Geometry: see drawing. Coordinates: mm, zero at the bounding-box minimum. Coordinates: 2 decimals unless noted, no trailing zeros. Loops run counter-clockwise (first coordinate to the right, second up) from the corner with the lowest first, then second, coordinate; pieces in that order, holes last. Notation, with made-up numbers: (68, -0.5) -> (88, -0.5) arc R30 ccw to (88, 22.5) -> close; hole circle Ø4 at (14.25, -19.75). An arc over 180 degrees is marked (long way). One line per item, written item: value. Start each with the question number.
Item 1: Section query C-C on x = 150. Return loops of the section in (y, z).
Item 2: Contact query for flat-ended pins moving along their axis: pin 1 Ø1.6 at (y, z) = (36, 2) entering from -X; pin 2 Ø2 at (y, z) = (31.5, 3.5) entering from +X; pin 3 Ø1.6 at (x, z) = (215.5, 1.5) entering from -Y; pin 4 Ø2 at (x, y) = (91, 52) entering from -Z. Output: stop coordinate, or through.
Item 3: Ray query, probe 1 along Y at (x, z) = (40, 1.1); probe 2 along X at (y, z) = (4.5, 5.1); probe 3 along X at (y, z) = (30, 1.65). Return the intervals inside material, ascending. Write a range as from..to.
Item 4: Section query B-B on x = 227.5. Return loops of the section in (y, z).
Item 5: Section query A-A on z = 2.65. Return loops of the section in (x, y) (3 decimals).
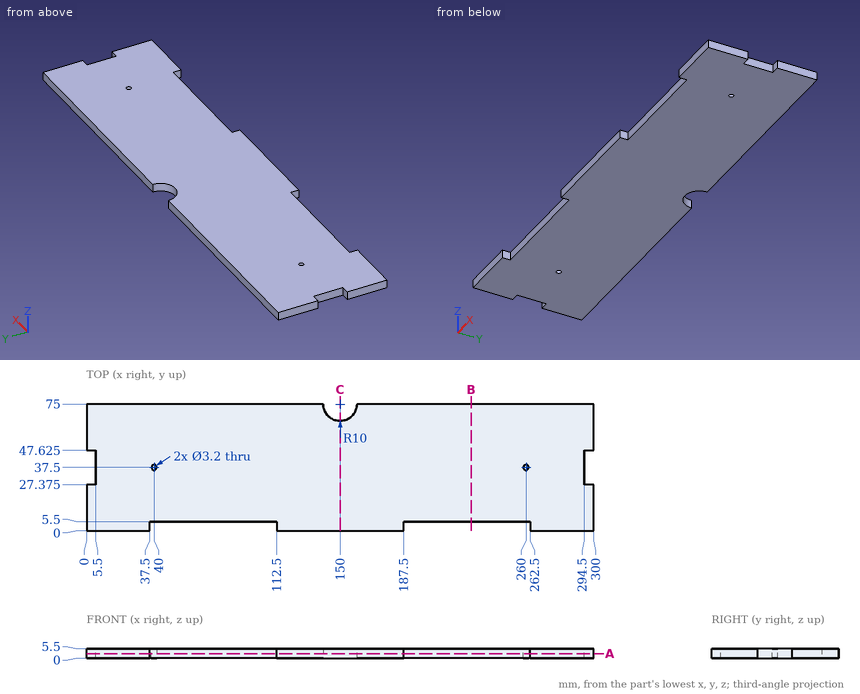
Reply:
1. outline: (0, 0) -> (65, 0) -> (65, 5.5) -> (0, 5.5) -> close
2. pin 1: stops at x = 5.5
2. pin 2: stops at x = 294.5
2. pin 3: stops at y = 5.5
2. pin 4: stops at z = 0
3. probe 1: y = 5.5..35.9, 39.1..75
3. probe 2: x = 0..37.5, 112.5..187.5, 262.5..300
3. probe 3: x = 5.5..294.5
4. outline: (5.5, 0) -> (75, 0) -> (75, 5.5) -> (5.5, 5.5) -> close
5. outline: (0, 0) -> (37.5, 0) -> (37.5, 5.5) -> (112.5, 5.5) -> (112.5, 0) -> (187.5, 0) -> (187.5, 5.5) -> (262.5, 5.5) -> (262.5, 0) -> (300, 0) -> (300, 27.375) -> (294.5, 27.375) -> (294.5, 47.625) -> (300, 47.625) -> (300, 75) -> (160, 75) arc R10 cw to (140, 75) -> (0, 75) -> (0, 47.625) -> (5.5, 47.625) -> (5.5, 27.375) -> (0, 27.375) -> close; hole circle Ø3.2 at (40, 37.5); hole circle Ø3.2 at (260, 37.5)
